Geometry: final body of the model. Coordinates: model frame, mm. Face numbers are marked on the shaded views. A direction names the side the tool comes from. Give positions to 0.01 mm unless a question says otherwise; leave off trailing zeros. Write each loop counter-clockwise with the first axis right and the second up, starting at its lowest first coordinate (ties: lowest second). Pieces come first, ordered by that corner, then holes. Notation, with made-up numbers: M 14,24.25 L 73,24.25 A12 cw 73,47.25 Z; hole C -36.75,46.25 d5. An arc over 180 degrees is marked long. Use a Markdown table: item, result. Add a question column.
1) Line query: line 1 (Y direction, x = 0, z = 10.5); line 2 (Z direction, x = -2.25, y = -6). Output: solid intervals per line, ascending.
2) Pin query (flat end, axial travel): pin 1 (4 mm diameter, centred on x = 0, y = 8, fed in from -Z); pin 2 (5.5 mm diameter, centred on x = 8, y = 0, fed in from +Z); pin 3 (1.5 mm diameter, centred on x = -5, z = 12, fed in from +Y); pin 4 (3 mm diameter, centred on x = -8, y = 0, fed in from +Z). Return the tip coordinate at first contact, or that it passes through.
3) Section A-A on y = 0. Return the cut outline in (x, z).
4) Section D-D on x = -8. Return the cut outline in (y, z), then the cut area to 3 significant figures.
5) Set-up query: the marked faces 5, 6 and 7. Return all of +Z, -Z, +X, -X, +Y, -Y with unobstructed straight access to the full face (end or side cutting, diameter ignored); none if empty.
6) Section C-C on z = 8.5. Return the cut outline in (x, y), then the cut area to 3 significant figures.
7) Draft query along Y for the marked faces 1, 2, 3 and 4. Return one class per face: +Y half, -Y half, draft (parallel to the pull), parting line (faces both ways), or undercut.
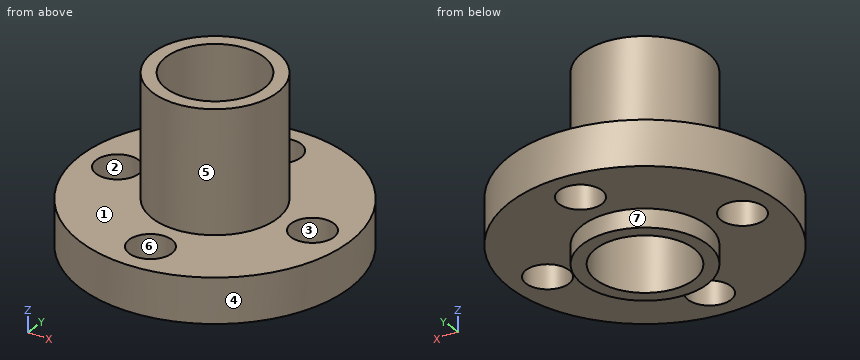
```python
from build123d import *

# Parameters (mm, degrees)
F_3_5_3_5_DIAMETER_HOLE1_D = 3.5


with BuildPart() as part:
    # Sketch1 → Revolve1 (revolve)
    with BuildSketch(Plane(origin=(0, 0, 0), x_dir=(1, 0, 0), z_dir=(0, 1, 0)), mode=Mode.PRIVATE) as revolve1_sk:
        Polygon((11, -1.5), (11, -5.15), (5.1, -5.15), (5.1, -15.05), (4, -15.05), (4, 0), (5.1, 0), (5.1, -1.5), align=None)
    revolve(revolve1_sk.sketch.rotate(Axis((0, 0, 0), (0, 0, 1)), 180), axis=Axis((0, 0, 0), (0, 0, 1)))

    # Ø3.5 (3.5) Diameter Hole1 (through all)
    with Locations(Plane.XY.offset(5.15)):
        with Locations((-8, 0), (0, 8), (8, 0), (0, -8)):
            Hole(F_3_5_3_5_DIAMETER_HOLE1_D / 2)


solid = part.part
```
Found:
| question | item | result |
|---|---|---|
| 1 | line 1 | -5.1 to -4, 4 to 5.1 |
| 1 | line 2 | 1.5 to 5.15 |
| 2 | pin 1 | z = 1.5 |
| 2 | pin 2 | z = 5.15 |
| 2 | pin 3 | y = 2.82 |
| 2 | pin 4 | through |
| 3 | outline | M -11,1.5 L -9.75,1.5 L -9.75,5.15 L -11,5.15 Z; M -6.25,1.5 L -5.1,1.5 L -5.1,0 L -4,0 L -4,15.05 L -5.1,15.05 L -5.1,5.15 L -6.25,5.15 Z; M 4,0 L 5.1,0 L 5.1,1.5 L 6.25,1.5 L 6.25,5.15 L 5.1,5.15 L 5.1,15.05 L 4,15.05 Z; M 9.75,1.5 L 11,1.5 L 11,5.15 L 9.75,5.15 Z |
| 4 | outline | M -7.55,1.5 L -1.75,1.5 L -1.75,5.15 L -7.55,5.15 Z; M 1.75,1.5 L 7.55,1.5 L 7.55,5.15 L 1.75,5.15 Z |
| 4 | area | 42.3 mm² |
| 5 | face 5 | +Z |
| 5 | face 6 | +Z, -Z |
| 5 | face 7 | -Z |
| 6 | outline | C 0,0 d10.2; hole C 0,0 d8 |
| 6 | area | 31.4 mm² |
| 7 | face 1 | draft |
| 7 | face 2 | undercut |
| 7 | face 3 | undercut |
| 7 | face 4 | parting line |
